Check sheet for the modelled part. Datum: model origin and axes. Units: mm. A direction names the side the tool comes from. Give positions to 0.01 mm unless a question says otherwise; leave off trailing zeros. Order: outer loops, then holes, each group sorted by start corner. A loop starts at its lowest first (then second) coordinate and runs counter-clockwise, first axis right, second up. Notation, with made-up numbers: (31.25, 51) -> (59.25, 51) arc R20 cw to (59.25, 79) -> close; hole circle Ø5 at (11.5, 61). An arc over 180 degrees is marked (long way). One line per question, with ' | ' between items.
```python
from build123d import *

# Parameters (mm, degrees)
SKETCH_1_R               = 20
EXTRUDE_1_DEPTH          = 20
SKETCH_2_R               = 10
EXTRUDE_2_DEPTH          = 33
SKETCH_4_W               = 21
SKETCH_4_H               = 21
SKETCH_4_W_2             = 17
SKETCH_4_H_2             = 17
CUT_EXTRUDE_3_DEPTH      = 15
CUT_EXTRUDE_4_DEPTH      = 61.074953184
CUT_EXTRUDE_4_DEPTH_BACK = 61.074953184
SKETCH_5_R               = 1.55
FILLET_1_R               = 10
CUT_EXTRUDE_6_DEPTH      = 20
CUT_EXTRUDE_7_DEPTH      = 62.522353742
CUT_EXTRUDE_7_DEPTH_BACK = 62.522353742
SKETCH_9_R               = 1.5


with BuildPart() as part:
    # 草图1 → 凸台-拉伸1 (new body)
    with BuildSketch(Plane.XY):
        Circle(SKETCH_1_R)
    extrude(amount=EXTRUDE_1_DEPTH)

    # 草图2 → 凸台-拉伸2 (add)
    with BuildSketch(Plane.XY.offset(20)):
        Circle(SKETCH_2_R)
    extrude(amount=EXTRUDE_2_DEPTH)

    # 草图4 → 切除-拉伸3 (cut)
    with BuildSketch(Plane(origin=(0, 0, 0), x_dir=(-1, 0, 0), z_dir=(0, 0, -1))):
        Rectangle(SKETCH_4_W, SKETCH_4_H)
        Rectangle(SKETCH_4_W_2, SKETCH_4_H_2, mode=Mode.SUBTRACT)
    extrude(amount=-CUT_EXTRUDE_3_DEPTH, mode=Mode.SUBTRACT)

    # 草图5 → 切除-拉伸4 (cut, two sides: drawn at the far end of the back side and taken through both)
    with BuildSketch(Plane(origin=(0, 0, 0), x_dir=(1, 0, 0), z_dir=(0, 1, 0)).offset(-CUT_EXTRUDE_4_DEPTH_BACK)):
        with Locations(Location((0, -10, 0), (0, 0, 270))):
            Circle(SKETCH_5_R)
    extrude(amount=CUT_EXTRUDE_4_DEPTH + CUT_EXTRUDE_4_DEPTH_BACK, mode=Mode.SUBTRACT)

    # 圆角1
    fillet_1_edges = [part.edges().sort_by_distance(p)[0] for p in [
        (-10, 0, 20),
    ]]
    fillet(fillet_1_edges, radius=FILLET_1_R - 0.0001)  # a hair under: the kernel refuses the full size

    # 草图8 → 切除-拉伸6 (cut)
    with BuildSketch(Plane.XY.offset(53)):
        with BuildLine():
            Line((-3.400367627, -4), (3.400367627, -4))
            ThreePointArc((3.400367627, -4), (0, 5.25), (-3.400367627, -4))
        make_face()
    extrude(amount=-CUT_EXTRUDE_6_DEPTH, mode=Mode.SUBTRACT)

    # 草图9 → 切除-拉伸7 (cut, two sides: drawn at the far end of the back side and taken through both)
    with BuildSketch(Plane(origin=(0, -4, 0), x_dir=(1, 0, 0), z_dir=(0, 1, 0)).offset(-CUT_EXTRUDE_7_DEPTH_BACK)):
        with Locations(Location((0, -43, 0), (0, 0, 180))):
            Circle(SKETCH_9_R)
    extrude(amount=CUT_EXTRUDE_7_DEPTH + CUT_EXTRUDE_7_DEPTH_BACK, mode=Mode.SUBTRACT)


solid = part.part
```
Q1. Section check D-D (z = 43). Enter the section's corners in (x, y).
Result sheet:
outline: (-3.4, -4) arc R5.25 cw to (-1.5, 5.03) -> (-1.5, 9.89) arc R10 ccw to (-1.5, -9.89) -> (-1.5, -4) -> close; (1.5, -9.89) arc R10 ccw to (1.5, 9.89) -> (1.5, 5.03) arc R5.25 cw to (3.4, -4) -> (1.5, -4) -> close
Q2. Section check C-C (x = 0). Count the separate pieces of the cut face and the enclosed holes in it, and give its area (3 significant figures).
Result sheet:
separate pieces: 6 | enclosed holes: 0 | area: 1,110 mm2
Q3. Thickness scan on line 1 (Y direction, x = 0, z = 45.25); line 2 (Y direction, x = 6.5, z = 11); line 3 (X direction, y = 6, z = 43). Record the ranges inside material, lowest first.
Result sheet:
line 1: y = -10 to -4, 5.25 to 10 | line 2: y = -18.91 to -10.5, -8.5 to 8.5, 10.5 to 18.91 | line 3: x = -8 to -1.5, 1.5 to 8
Q4. Section check A-A (z = 10). Enter the section's corners in (x, y).
Result sheet:
outline: (-10.5, -10.5) -> (-10.5, 10.5) -> (-1.55, 10.5) -> (-1.55, 19.94) arc R20 ccw to (-1.55, -19.94) -> (-1.55, -10.5) -> close; (-8.5, -8.5) -> (-1.55, -8.5) -> (-1.55, 8.5) -> (-8.5, 8.5) -> close; (1.55, -19.94) arc R20 ccw to (1.55, 19.94) -> (1.55, 10.5) -> (10.5, 10.5) -> (10.5, -10.5) -> (1.55, -10.5) -> close; (1.55, -8.5) -> (8.5, -8.5) -> (8.5, 8.5) -> (1.55, 8.5) -> close
Q5. Mould release check, pull along Z, two halves, no side actions. Record for faces 4 (the face through (-0.94, -15.32, 8.77)), 5 (the face through (0, 1, 33)), 6 (the face through (0, -10.5, 7)): pulls with the +Z half, pulls with the -Z half, needs draft (parallel to the pull), parting line crosses it, or undercut.
Result sheet:
face 4: undercut | face 5: pulls with the +Z half | face 6: needs draft
Q6. Access from +Z, -Z, +X, -X, +Y, -Y to the whole of each face (thin tool, end or side, straight path). Record for faces 1 (the face through (10.5, 0, 7)), 2 (the face through (-4.336, -19.524, 9.86)), 3 (the face through (-2, -4, 43)).
Result sheet:
face 1: -Z | face 2: +Z, -Z | face 3: +Z
Q7. Depth check by flat-ended pin: pin 1 Ø3 at (x, z) = (0, 10) entering from +Y; pin 2 Ø7.5 at (x, z) = (4.5, 11) entering from +Y; pin 3 Ø5 at (x, z) = (0, 43) entering from -Y; pin 4 Ø1.5 at (y, z) = (-3.5, 11.5) entering from +X. Enter the tip coordinate at first touch or a pass-through.
Result sheet:
pin 1: passes through | pin 2: stops at y = 19.99 | pin 3: stops at y = -10 | pin 4: stops at x = 19.81
